from build123d import *

# Parameters (mm, degrees)
SKETCH2_W           = 55
SKETCH2_H           = 55
SKETCH2_W_2         = 30
SKETCH2_H_2         = 30
BOSS_EXTRUDE1_DEPTH = 35
SKETCH3_W           = 55
SKETCH3_H           = 55
SKETCH3_R           = 3.2
BOSS_EXTRUDE2_DEPTH = 2.5
SKETCH4_W           = 55
SKETCH4_H           = 55
SKETCH4_R           = 3.2
BOSS_EXTRUDE3_DEPTH = 2.5
SKETCH6_R           = 18.2
SKETCH6_R_2         = 3.2
BOSS_EXTRUDE4_DEPTH = 1
SKETCH7_W           = 15
SKETCH7_H           = 23
BOSS_EXTRUDE5_DEPTH = 10
CHAMFER1_SIZE       = 3
SKETCH8_W           = 10
SKETCH8_H           = 10
CUT_EXTRUDE1_DEPTH  = 70
SKETCH9_R           = 2
CUT_EXTRUDE2_DEPTH  = 5


with BuildPart() as part:
    # Sketch2 → Boss-Extrude1 (new body, symmetric)
    with BuildSketch(Plane.XY):
        Rectangle(SKETCH2_W, SKETCH2_H)
        Rectangle(SKETCH2_W_2, SKETCH2_H_2, mode=Mode.SUBTRACT)
    extrude(amount=BOSS_EXTRUDE1_DEPTH, both=True)

    # Sketch3 → Boss-Extrude2 (add)
    with BuildSketch(Plane.XY.offset(35)):
        Rectangle(SKETCH3_W, SKETCH3_H)
        Circle(SKETCH3_R, mode=Mode.SUBTRACT)
    extrude(amount=BOSS_EXTRUDE2_DEPTH)

    # Sketch4 → Boss-Extrude3 (add)
    with BuildSketch(Plane(origin=(0, 0, -35), x_dir=(-1, 0, 0), z_dir=(0, 0, -1))):
        Rectangle(SKETCH4_W, SKETCH4_H)
        Circle(SKETCH4_R, mode=Mode.SUBTRACT)
    extrude(amount=BOSS_EXTRUDE3_DEPTH)

    # Sketch6 → Boss-Extrude4 (add)
    with BuildSketch(Plane.XY.offset(37.5)):
        Circle(SKETCH6_R)
        Circle(SKETCH6_R_2, mode=Mode.SUBTRACT)
    extrude(amount=BOSS_EXTRUDE4_DEPTH)

    # Sketch7 → Boss-Extrude5 (add)
    with BuildSketch(Plane(origin=(27.5, 0, 0), x_dir=(0, 0, -1), z_dir=(1, 0, 0))):
        with Locations((30, 0)):
            Rectangle(SKETCH7_W, SKETCH7_H)
    extrude(amount=BOSS_EXTRUDE5_DEPTH)

    # Chamfer1
    chamfer1_edges = [part.edges().sort_by_distance(p)[0] for p in [
        (37.5, 0, -22.5),
        (37.5, -11.5, -30),
        (37.5, 0, -37.5),
        (37.5, 11.5, -30),
    ]]
    chamfer(chamfer1_edges, length=CHAMFER1_SIZE)

    # Sketch8 → Cut-Extrude1 (cut)
    with BuildSketch(Plane(origin=(0, 0, -37.5), x_dir=(-1, 0, 0), z_dir=(0, 0, -1))):
        with Locations((-22.5, 22.5)):
            Rectangle(SKETCH8_W, SKETCH8_H)
        with Locations((22.5, 22.5)):
            Rectangle(SKETCH8_W, SKETCH8_H)
        with Locations((-22.5, -22.5)):
            Rectangle(SKETCH8_W, SKETCH8_H)
        with Locations((22.5, -22.5)):
            Rectangle(SKETCH8_W, SKETCH8_H)
    extrude(amount=-CUT_EXTRUDE1_DEPTH, mode=Mode.SUBTRACT)

    # Sketch9 → Cut-Extrude2 (cut)
    with BuildSketch(Plane.XY.offset(37.5)):
        with Locations((-22.5, 22.5)):
            Circle(SKETCH9_R)
        with Locations((22.5, 22.5)):
            Circle(SKETCH9_R)
        with Locations((-22.5, -22.5)):
            Circle(SKETCH9_R)
        with Locations((22.5, -22.5)):
            Circle(SKETCH9_R)
    extrude(amount=-CUT_EXTRUDE2_DEPTH, mode=Mode.SUBTRACT)


solid = part.part
Geometry: final body of the model. Coordinates: model frame, mm. A direction names the side the tool comes from. Round coordinates to 2 decimals unless told otherwise and drop trailing zeros. Loops run counter-clockwise (first coordinate to the right, second up) from the corner with the lowest first, then second, coordinate; pieces in that order, holes last.
Q1. Pull-direction query (Z, two-part tool) for faces 1 (the flat face through (-20, -22, 32.5)), 2 (the flat face through (4, 0, -35)), 3 (the flat face through (0, -4, 38.5)), 4 (the flat face through (0, 27.5, 1)); classes: released by +Z, released by -Z, zero draft, split by the parting line, or undercut.
Q2. Section C-C on x = 0. Return loops of the section in (y, z), plus the area to 3 significant figures.
Q3. Section A-A on x = -22.5. Return loops of the section in (y, z).
Q4. Access query for faces 5 (the flat face through (23, -17.5, -3)), 6 (the flat face through (31, -11.5, -30)), 7 (the flat face through (-19, 0, 37.5)), 8 (the flat face through (25, 23, 32.5)). Directions: +Z, -Z, +X, -X, +Y, -Y. A direction counts if a zero-diameter tool reaches every point of the face in a straight line with its end or side. Return the directions, or none.
Q5. Material intervals for L1, parallel to Y at x = 14.5, z = -31.5; L2, parallel to Y at x = 22.5, z = 34, sorted ascending.
Q6. Section B-B on y = 0. Return loops of the section in (x, z).
Q7. Pin query (flat end, axial travel): P1, Ø6, axis at x = 22.5, z = -3, coming from the +Y side; P2, Ø5.5, axis at x = 32, z = -32.5, coming from the -Y side; P3, Ø6.5, axis at x = 22.5, y = -22.5, coming from the -Z side. Return the tip coordinate at first contact, or that it passes through.
Evaluation:
1. face 1: released by -Z
1. face 2: undercut
1. face 3: released by +Z
1. face 4: zero draft
2. outline: (-27.5, -37.5) - (-3.2, -37.5) - (-3.2, -35) - (-15, -35) - (-15, 35) - (-3.2, 35) - (-3.2, 38.5) - (-18.2, 38.5) - (-18.2, 37.5) - (-27.5, 37.5) - close; (3.2, -37.5) - (27.5, -37.5) - (27.5, 37.5) - (18.2, 37.5) - (18.2, 38.5) - (3.2, 38.5) - (3.2, 35) - (15, 35) - (15, -35) - (3.2, -35) - close
2. area: 2,020 mm2
3. outline: (-27.5, 32.5) - (-24.5, 32.5) - (-24.5, 37.5) - (-27.5, 37.5) - close; (-20.5, 32.5) - (-17.5, 32.5) - (-17.5, -37.5) - (17.5, -37.5) - (17.5, 32.5) - (20.5, 32.5) - (20.5, 37.5) - (-20.5, 37.5) - close; (24.5, 32.5) - (27.5, 32.5) - (27.5, 37.5) - (24.5, 37.5) - close
4. face 5: -Z, +X, -Y
4. face 6: +Z, -Z, +X, -Y
4. face 7: +Z
4. face 8: -Z, +X, +Y
5. L1: y = -27.5 to -15, 15 to 27.5
5. L2: y = -27.5 to -24.5, -20.5 to 20.5, 24.5 to 27.5
6. outline: (-27.5, -37.5) - (-3.2, -37.5) - (-3.2, -35) - (-15, -35) - (-15, 35) - (-3.2, 35) - (-3.2, 38.5) - (-18.2, 38.5) - (-18.2, 37.5) - (-27.5, 37.5) - close; (3.2, -37.5) - (34.5, -37.5) - (37.5, -34.5) - (37.5, -25.5) - (34.5, -22.5) - (27.5, -22.5) - (27.5, 37.5) - (18.2, 37.5) - (18.2, 38.5) - (3.2, 38.5) - (3.2, 35) - (15, 35) - (15, -35) - (3.2, -35) - close
7. P1: stops at y = 17.5
7. P2: stops at y = -11.5
7. P3: stops at z = 32.5
